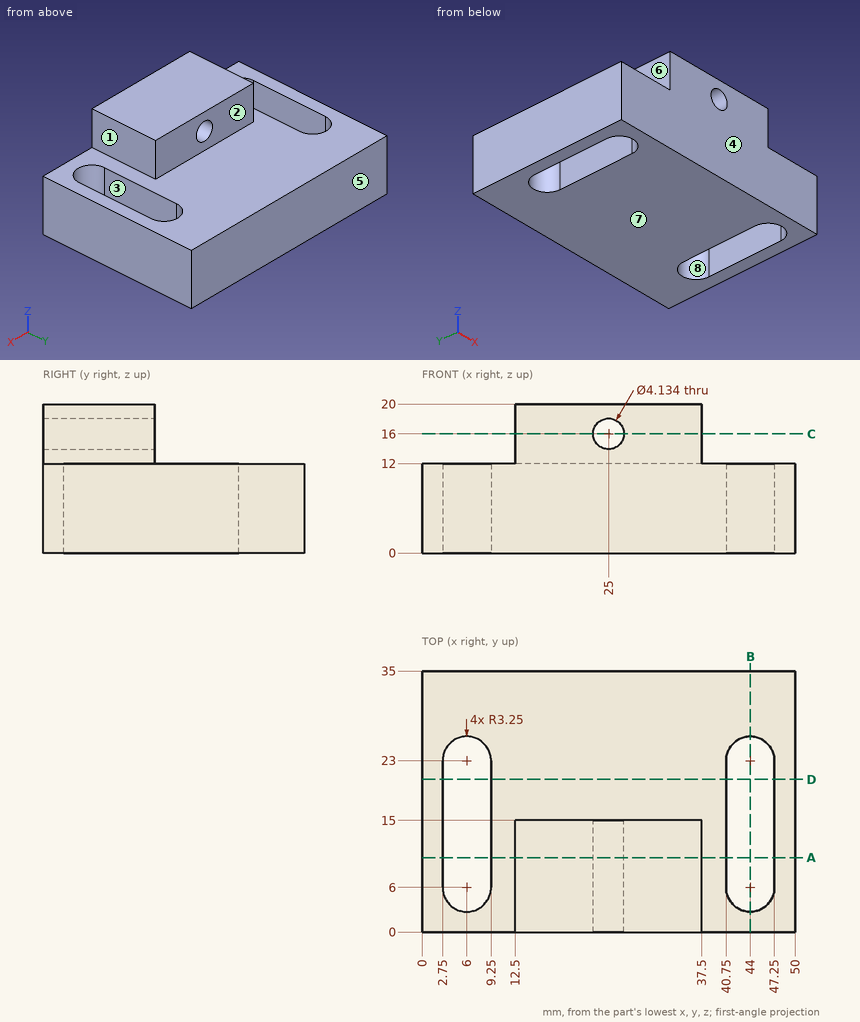
The figure shows three views and two pictorial views of one solid part (mm, origin at its lowest corner). Answer the questions. A direction names the side the tool comes from. Coordinates: 2 decimals unless noted, no trailing zeros. Write each loop counter-clockwise with the first axis right and the second up, starting at its lowest first coordinate (ties: lowest second). Pieces come first, ordered by that corner, then holes. Notation, with made-up numbers: (17, 64) -> (42, 64) arc R23 ccw to (42, 77) -> close; hole circle Ø11 at (58, -6). An arc over 180 degrees is marked (long way). Return JSON: item names as keys, results as strings.
1. Find the intervals of material crossed by line 1 along X through (y, z) = (25, 8); line 2 along Y through (x, z) = (44, 1.25); line 3 along X through (y, z) = (8, 8.5), in increasing order. Write a range as from..to.
Found:
{"line 1": "0..3.44, 8.56..41.44, 46.56..50", "line 2": "0..2.75, 26.25..35", "line 3": "0..2.75, 9.25..40.75, 47.25..50"}
2. Determine the mould class of the marked faces 6, 7 and 8 for opening direction X: pulls with the +X half, pulls with the -X half, needs draft (parallel to the pull), parting line crosses it, or undercut.
Found:
{"face 6": "pulls with the -X half", "face 7": "needs draft", "face 8": "undercut"}
3. A cutting plane is placed at D-D (y = 20.5). Determine the outline of the cut face in (x, z), and give its area (3 significant figures).
Found:
{"outline": "(0, 0) -> (2.75, 0) -> (2.75, 12) -> (0, 12) -> close; (9.25, 0) -> (40.75, 0) -> (40.75, 12) -> (9.25, 12) -> close; (47.25, 0) -> (50, 0) -> (50, 12) -> (47.25, 12) -> close", "area": "444 mm2"}
4. Each of these flat-tipped pins is pushed along its axis until it touches: P1, Ø10, axis at x = 37, z = 16.5, coming from the -Y side; P2, Ø4, axis at y = 5, z = 17.5, coming from the -X side; P3, Ø10.5, axis at x = 28.5, y = 21.5, coming from the +Z side; P4, Ø4, axis at y = 11, z = 16.5, coming from the +X side. Where does it stop, or does it pass through?
Found:
{"P1": "y = 0", "P2": "x = 12.5", "P3": "z = 12", "P4": "x = 37.5"}
5. A tool of negligible diameter and unlimited length cuts with its end or side. For the marked faces 1, 2, 3, 4 and 5, from which of +Z, -Z, +X, -X, +Y, -Y can it reach the whole face along a straight path? Write none if from no direction.
Found:
{"face 1": "+Z, +X, +Y, -Y", "face 2": "+Z, +X, -X, +Y", "face 3": "+Z, -Z", "face 4": "+Z, -Z, +X, -X, -Y", "face 5": "+Z, -Z, +X, -X, +Y"}
6. A cutting plane is placed at A-A (y = 10). Determine the outline of the cut face in (x, z), and give its area (3 significant figures).
Found:
{"outline": "(0, 0) -> (2.75, 0) -> (2.75, 12) -> (0, 12) -> close; (9.25, 0) -> (40.75, 0) -> (40.75, 12) -> (37.5, 12) -> (37.5, 20) -> (12.5, 20) -> (12.5, 12) -> (9.25, 12) -> close; (47.25, 0) -> (50, 0) -> (50, 12) -> (47.25, 12) -> close; hole circle Ø4.13 at (25, 16)", "area": "631 mm2"}
7. A cutting plane is placed at B-B (x = 44). Determine the outline of the cut face in (y, z).
Found:
{"outline": "(0, 0) -> (2.75, 0) -> (2.75, 12) -> (0, 12) -> close; (26.25, 0) -> (35, 0) -> (35, 12) -> (26.25, 12) -> close"}
8. A cutting plane is placed at C-C (z = 16). Determine the outline of the cut face in (x, y).
Found:
{"outline": "(12.5, 0) -> (22.93, 0) -> (22.93, 15) -> (12.5, 15) -> close; (27.07, 0) -> (37.5, 0) -> (37.5, 15) -> (27.07, 15) -> close"}
